For this review, use the dimensioned drawing (mm, ordinates from the lowest corner) and the shaded views. Give positions to 0.01 mm unless a question says otherwise; leave off trailing zeros. Loops run counter-clockwise (first coordinate to the right, second up) from the corner with the lowest first, then second, coordinate; pieces in that order, holes last. Notation, with made-up numbers: M 67,15.25 L 105,15.25 A10 ccw 105,26.25 Z; hole C -36,71.5 d6. An arc over 180 degrees is marked long. Return JSON: item names as keys, results as strings.
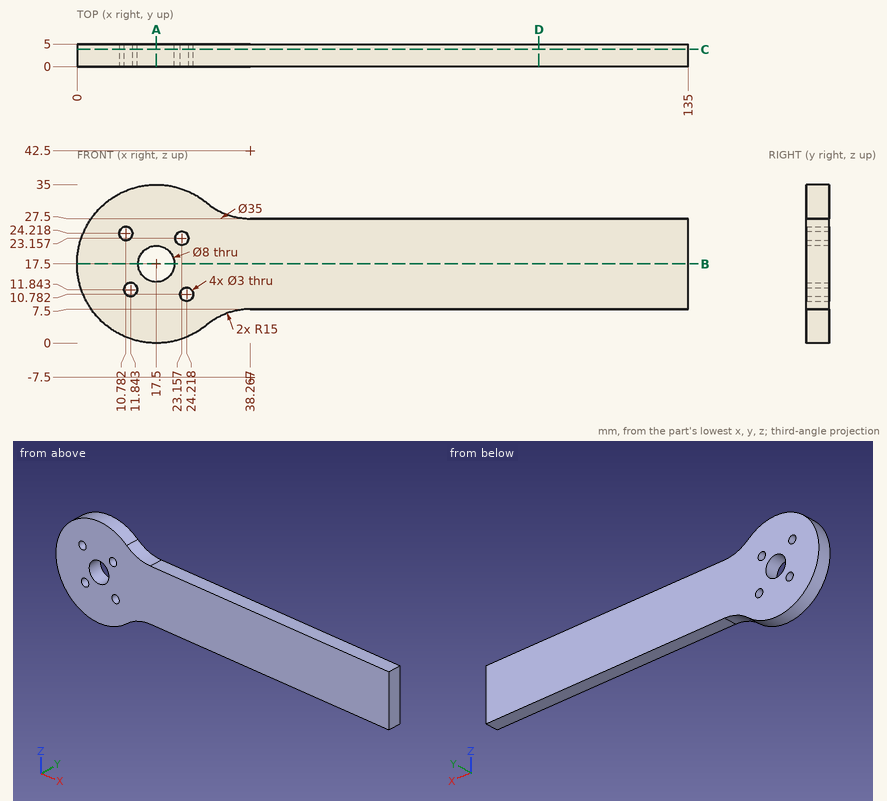
1) Consider section C-C on y = 3.8. Write out the cut boundary in (x, z).
From the geometry:
{"outline": "M 28.68,4.04 A15 cw 38.27,7.5 L 135,7.5 L 135,27.5 L 38.27,27.5 A15 cw 28.68,30.96 A17.5 ccw long Z; hole C 10.78,24.22 d3; hole C 11.84,11.84 d3; hole C 17.5,17.5 d8; hole C 23.16,23.16 d3; hole C 24.22,10.78 d3"}
2) Consider section B-B on z = 17.5. Write out the cut boundary in (x, y).
From the geometry:
{"outline": "M 0,0 L 13.5,0 L 13.5,5 L 0,5 Z; M 21.5,0 L 135,0 L 135,5 L 21.5,5 Z"}
3) Wall thickness on L1, parallel to X at y = 1.1, z = 24.5 (1 decimal); L2, parallel to Z at x = 114.5, y = 1; L3, parallel to X at y = 3.2, z = 17.5: over which ranges is each line inside the solid? List them lowest first. Write a range as from..to.
From the geometry:
{"L1": "1.5..9.3, 12.3..22.5, 23.8..135", "L2": "7.5..27.5", "L3": "0..13.5, 21.5..135"}
4) Insertion check: pin 1 (3 mm diameter, centred on x = 53.5, z = 29.5, fed in from +Y); pin 2 (1 mm diameter, centred on x = 14.5, y = 0.5, fed in from -Z). Each pin has a flat end and moves straight along its axis. Give the tip position at first contact, or say it passes through.
From the geometry:
{"pin 1": "through", "pin 2": "z = 0.18"}
5) Consider section A-A on x = 17.5. Write out the cut boundary in (y, z), then the cut area to 3 significant figures.
From the geometry:
{"outline": "M 0,0 L 5,0 L 5,13.5 L 0,13.5 Z; M 0,21.5 L 5,21.5 L 5,35 L 0,35 Z", "area": "135 mm²"}
6) Consider section D-D on x = 102. Write out the cut boundary in (y, z), then the cut area to 3 significant figures.
From the geometry:
{"outline": "M 0,7.5 L 5,7.5 L 5,27.5 L 0,27.5 Z", "area": "100 mm²"}
